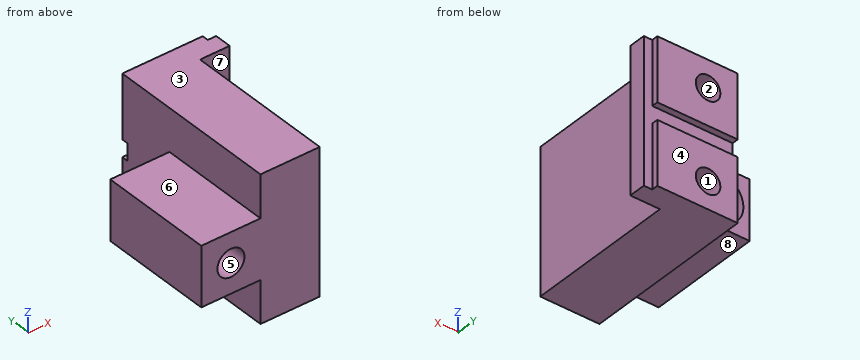
from build123d import *

# Parameters (mm, degrees)
SALIENTE_EXTRUIR1_DEPTH      = 7
CROQUIS5_R                   = 1.6
CORTAR_EXTRUIR2_DEPTH        = 13.9
CROQUIS6_R                   = 2.75
CORTAR_EXTRUIR3_DEPTH        = 3
SALIENTE_EXTRUIR2_DEPTH      = 5
SALIENTE_EXTRUIR2_DEPTH_BACK = 12
CROQUIS8_R                   = 1.45
CORTAR_EXTRUIR4_DEPTH        = 10
CROQUIS9_W                   = 2
CROQUIS9_H                   = 0.75
CORTAR_EXTRUIR5_DEPTH        = 10
CROQUIS10_R                  = 1.6
SALIENTE_EXTRUIR3_DEPTH      = 4


with BuildPart() as part:
    # Croquis1 → Saliente-Extruir1 (new body)
    with BuildSketch(Plane.XY):
        Polygon((0, 0), (4, 0), (4, -4), (7, -4), (7, 0), (7, 13.75), (10.5, 13.75), (10.5, 15.75), (9.5, 15.75), (9.5, 16.5), (7, 16.5), (0, 16.5), (0, 9.5), (-7, 9.5), (-7, 0), align=None)
    extrude(amount=SALIENTE_EXTRUIR1_DEPTH)

    # Croquis5 → Cortar-Extruir2 (cut)
    with BuildSketch(Plane(origin=(0, 9.5, 0), x_dir=(1, 0, 0), z_dir=(0, 1, 0))):
        with Locations(Location((-3.5, -3.5, 0), (0, 0, 180))):
            Circle(CROQUIS5_R)
    extrude(amount=-CORTAR_EXTRUIR2_DEPTH, mode=Mode.SUBTRACT)

    # Croquis6 → Cortar-Extruir3 (cut)
    with BuildSketch(Plane(origin=(0, 9.5, 0), x_dir=(1, 0, 0), z_dir=(0, 1, 0))):
        with Locations(Location((-3.5, -3.5, 0), (0, 0, 180))):
            Circle(CROQUIS6_R)
    extrude(amount=-CORTAR_EXTRUIR3_DEPTH, mode=Mode.SUBTRACT)

    # Croquis7 → Saliente-Extruir2 (add, two sides: drawn at the far end of the back side and taken through both)
    with BuildSketch(Plane.XY.offset(7).offset(-SALIENTE_EXTRUIR2_DEPTH_BACK)):
        Polygon((0, 16.5), (0, 0), (7, 0), (7, 13.75), (10.5, 13.75), (10.5, 15.75), (9.5, 15.75), (9.5, 16.5), align=None)
    extrude(amount=SALIENTE_EXTRUIR2_DEPTH + SALIENTE_EXTRUIR2_DEPTH_BACK)

    # Croquis8 → Cortar-Extruir4 (cut)
    with BuildSketch(Plane(origin=(0, 16.5, 0), x_dir=(1, 0, 0), z_dir=(0, 1, 0))):
        with Locations(Location((3.5, 1.8, 0), (0, 0, 270))):
            Circle(CROQUIS8_R)
        with Locations(Location((3.5, -8.8, 0), (0, 0, 90))):
            Circle(CROQUIS8_R)
    extrude(amount=-CORTAR_EXTRUIR4_DEPTH, mode=Mode.SUBTRACT)

    # Croquis9 → Cortar-Extruir5 (cut)
    with BuildSketch(Plane(origin=(9.5, 0, 0), x_dir=(0, 0, -1), z_dir=(1, 0, 0))):
        with Locations((-3.5, 16.125)):
            Rectangle(CROQUIS9_W, CROQUIS9_H)
    extrude(amount=-CORTAR_EXTRUIR5_DEPTH, mode=Mode.SUBTRACT)

    # Croquis10 → Saliente-Extruir3 (add)
    with BuildSketch(Plane.XZ):
        Polygon((-7, 0), (0, 0), (0, -5), (7, -5), (7, 0), (4, 0), (4, 7), (7, 7), (7, 12), (0, 12), (0, 7), (-7, 7), align=None)
        with Locations(Location((-3.5, 3.5, 0), (0, 0, 180))):
            Circle(CROQUIS10_R, mode=Mode.SUBTRACT)
    extrude(amount=SALIENTE_EXTRUIR3_DEPTH)


solid = part.part
Verification items for the finished model (mm, model axes). Face numbers are marked on the shaded views. A direction names the side the tool comes from. Give positions to 0.01 mm unless a question says otherwise; leave off trailing zeros. Loops run counter-clockwise (first coordinate to the right, second up) from the corner with the lowest first, then second, coordinate; pieces in that order, holes last.
1. Release check for a two-part mould opening along Z. For the marked faces 1, 2, 3 and 4 record: +Z half, -Z half, draft (parallel to the pull), parting line (faces both ways), or undercut.
Derived:
face 1: undercut
face 2: undercut
face 3: +Z half
face 4: draft
2. Cross-section at B-B on x = 3.5. Record the cut outline in (y, z), and give its area (3 significant figures).
Derived:
outline: (-4, -5) - (16.5, -5) - (16.5, -3.25) - (6.5, -3.25) - (6.5, -0.35) - (16.5, -0.35) - (16.5, 2.5) - (15.75, 2.5) - (15.75, 4.5) - (16.5, 4.5) - (16.5, 7.35) - (6.5, 7.35) - (6.5, 10.25) - (16.5, 10.25) - (16.5, 12) - (-4, 12) - close
area: 289 mm2
3. Material ranges on probe 1 along X at (y, z) = (2.25, 3.5); probe 2 along Z at (x, y) = (-3.5, 8.65); probe 3 along Z at (x, y) = (4.25, 7), recorded low to high.
Derived:
probe 1: x = -7 to -5.1, -1.9 to 7
probe 2: z = 0 to 0.75, 6.25 to 7
probe 3: z = -5 to -3.04, -0.56 to 7.56, 10.04 to 12
4. Go/stop test with flat-tipped pins: P1, Ø8.5, axis at x = 3, z = 4, coming from the +Y side; P2, Ø1.4, axis at x = 3.5, z = 9.5, coming from the +Y side; P3, Ø6, axis at x = -4, z = 2.5, coming from the +Y side; P4, Ø1.5, axis at y = 7, z = 0, coming from the +X side. Record where each tip stops, or that it passes through.
Derived:
P1: stops at y = 16.5
P2: stops at y = 6.5
P3: stops at y = 9.5
P4: stops at x = 7
5. Cross-section at A-A on z = 3.5. Record the cut outline in (x, y).
Derived:
outline: (-7, -4) - (-5.1, -4) - (-5.1, 6.5) - (-6.25, 6.5) - (-6.25, 9.5) - (-7, 9.5) - close; (-1.9, -4) - (7, -4) - (7, 13.75) - (10.5, 13.75) - (10.5, 15.75) - (0, 15.75) - (0, 9.5) - (-0.75, 9.5) - (-0.75, 6.5) - (-1.9, 6.5) - close
6. Cross-section at D-D on z = -1.8. Record the cut outline in (x, y).
Derived:
outline: (0, -4) - (7, -4) - (7, 13.75) - (10.5, 13.75) - (10.5, 15.75) - (9.5, 15.75) - (9.5, 16.5) - (4.95, 16.5) - (4.95, 6.5) - (2.05, 6.5) - (2.05, 16.5) - (0, 16.5) - close
7. Cross-section at C-C on y = 5. Record the cut outline in (x, z).
Derived:
outline: (-7, 0) - (0, 0) - (0, -5) - (7, -5) - (7, 12) - (0, 12) - (0, 7) - (-7, 7) - close; hole circle Ø3.2 at (-3.5, 3.5)
8. Tool access check on the marked faces 5, 6, 7 and 8. Record the directions out of +Z, -Z, +X, -X, +Y, -Y that give a thin tool (end or side, any length) a straight path to the whole face; none if there is none.
Derived:
face 5: +Y, -Y
face 6: +Z, -X, +Y, -Y
face 7: +Z, -Z, +X, -Y
face 8: -Z, -X, +Y, -Y
